```python
from build123d import *

# Parameters (mm, degrees)
F1_DEPTH = 10
F2_DEPTH = 30
F4_DEPTH = 75.001
F6_DEPTH = 55.001


with BuildPart() as f1:
    # F0 (on Front) → F1 (new body)
    with BuildSketch(Plane.XZ):
        Polygon((50, 37.368118), (0, 37.368118), (-50, 37.368118), (-50, -12.631882), (-40, -22.631882), (-25, -22.631882), (-25, 32.368118), (25, 32.368118), (25, -22.631882), (40, -22.631882), (50, -12.631882), align=None)
    extrude(amount=F1_DEPTH)

    # F0 (on Front) → F2 (join)
    with BuildSketch(Plane.XZ):
        Polygon((-25, 32.368118), (-25, -22.631882), (0, -22.631882), (25, -22.631882), (25, 32.368118), align=None)
    extrude(amount=F2_DEPTH)

    # F3 (on face) → F4 (cut, through all)
    with BuildSketch(Plane.YZ.offset(25)):
        Polygon((-25, 32.368118), (-30, 32.368118), (-30, 27.368118), (-29.947912, 27.368118), (-25, 27.368118), align=None)
        with BuildLine():
            Line((-29.947912, 27.368118), (-30, 27.368118))
            Line((-30, 27.368118), (-30, -22.631882))
            Line((-30, -22.631882), (-10, -22.631882))
            ThreePointArc((-10, -22.631882), (-24.305881, 0.639861), (-29.947912, 27.368118))
        make_face()
    extrude(amount=-F4_DEPTH, mode=Mode.SUBTRACT)

    # F5 (on face) → F6 (cut, through all)
    with BuildSketch(Plane.XY.offset(32.368118)):
        Polygon((-14.46383, -25), (14.46383, -25), (8.660254, -14.947912), (-8.660254, -14.947912), align=None)
        Polygon((17.320508, -29.947912), (14.46383, -25), (-14.46383, -25), (-17.320508, -29.947912), (0, -29.947912), align=None)
    extrude(amount=-F6_DEPTH, mode=Mode.SUBTRACT)


solid = f1.part
```
Verification items for the finished model (mm, model axes). A direction names the side the tool comes from. Round coordinates to 2 decimals unless told otherwise and drop trailing zeros. Write each loop counter-clockwise with the first axis right and the second up, starting at its lowest first coordinate (ties: lowest second). Pieces come first, ordered by that corner, then holes.
1. Section check A-A on y = -19.25. Enter the section's corners in (x, z), plus the area to 3 significant figures.
2. Section check C-C on x = -20.5. Enter the section's corners in (y, z).
3. Draft check along X on faces 1 (the flat face through (0, -14.948, 8)), 2 (the flat face through (-1, 0, 8)), 3 (the flat face through (25, -18, 11)). Enter one of: +X half, -X half, draft (parallel to the pull), parting line (faces both ways), or undercut.
4. Access from +Z, -Z, +X, -X, +Y, -Y to the whole of each face (thin tool, end or side, straight path). Record for faces 4 (the flat face through (-25, -18, 11)), 5 (the flat face through (-21, -28, 27.368)), 6 (the flat face through (-50, -5, 13)).
5. Section check B-B on z = 29. Enter the section's corners in (x, y), plus the area to 3 significant figures.
6. Scan lines: L1, parallel to X at y = -13, z = 23.5; L2, parallel to X at y = -15.75, z = 26.5; L3, parallel to X at y = -17.25, z = -4. Record each from-to range of solid material in increasing order.
7. Gauge pin test, flat ends, axial feed: P1, Ø16, axis at y = -24.5, z = 17, coming from the +X side; P2, Ø1.5, axis at x = -19.5, z = 30.5, coming from the -Y side; P3, Ø1.5, axis at x = -18, y = -27.5, coming from the +Z side. Record the tip position at first contact, or that the pin passes through.
8. Section check D-D on y = -7. Enter the section's corners in (x, z), plus the area to 3 significant figures.
Answer:
1. outline: (-25, -9.77) - (-11.14, -9.77) - (-11.14, 32.37) - (-25, 32.37) - close; (11.14, -9.77) - (25, -9.77) - (25, 32.37) - (11.14, 32.37) - close
1. area: 1,170 mm2
2. outline: (-29.95, 27.37) arc R80 ccw to (-10, -22.63) - (0, -22.63) - (0, 37.37) - (-10, 37.37) - (-10, 32.37) - (-25, 32.37) - (-25, 27.37) - close
3. face 1: undercut
3. face 2: draft
3. face 3: +X half
4. face 4: +Z, -Z, -X, -Y
4. face 5: +Z, +X, -X, -Y
4. face 6: +Z, -Z, -X, +Y, -Y
5. outline: (-50, -10) - (-25, -10) - (-25, -25) - (-14.46, -25) - (-8.66, -14.95) - (8.66, -14.95) - (14.46, -25) - (25, -25) - (25, -10) - (50, -10) - (50, 0) - (-50, 0) - close
5. area: 1,520 mm2
6. L1: x = -25 to 25
6. L2: x = -25 to -9.12, 9.12 to 25
6. L3: x = -25 to -9.99, 9.99 to 25
7. P1: stops at x = 25
7. P2: stops at y = -25
7. P3: stops at z = 27.37
8. outline: (-50, -12.63) - (-40, -22.63) - (40, -22.63) - (50, -12.63) - (50, 37.37) - (-50, 37.37) - close
8. area: 5,900 mm2
